from build123d import *

# Parameters (mm, degrees)
SKETCH1_W                = 188
SKETCH1_H                = 90
SKETCH1_R                = 3
BOSS_EXTRUDE1_DEPTH      = 2
BOSS_EXTRUDE2_DEPTH      = 31.5
BOSS_EXTRUDE2_DEPTH_BACK = 7
SKETCH2_W                = 14
SKETCH2_H                = 37


with BuildPart() as part:
    # Sketch1 → Boss-Extrude1 (new body)
    with BuildSketch(Plane(origin=(0, 0, 0), x_dir=(1, 0, 0), z_dir=(0, 1, 0))):
        Rectangle(SKETCH1_W, SKETCH1_H)
        with Locations(Location((-89, 37.75, 0), (0, 0, 270))):
            Circle(SKETCH1_R, mode=Mode.SUBTRACT)
        with Locations(Location((89, 37.75, 0), (0, 0, 270))):
            Circle(SKETCH1_R, mode=Mode.SUBTRACT)
        with Locations(Location((89, -37.75, 0), (0, 0, 270))):
            Circle(SKETCH1_R, mode=Mode.SUBTRACT)
        with Locations(Location((-89, -37.75, 0), (0, 0, 270))):
            Circle(SKETCH1_R, mode=Mode.SUBTRACT)
    extrude(amount=BOSS_EXTRUDE1_DEPTH)

    # Sketch2 → Boss-Extrude2 (add, two sides: drawn at the far end of the back side and taken through both)
    with BuildSketch(Plane(origin=(0, 2, 0), x_dir=(1, 0, 0), z_dir=(0, 1, 0)).offset(-BOSS_EXTRUDE2_DEPTH_BACK)):
        Polygon((-80, -28), (-80, -45), (80, -45), (80, 45), (-80, 45), (-80, 9), align=None)
        with Locations((-87, -9.5)):
            Rectangle(SKETCH2_W, SKETCH2_H)
    extrude(amount=BOSS_EXTRUDE2_DEPTH + BOSS_EXTRUDE2_DEPTH_BACK)


solid = part.part
CAD build for the part. Positions are in the model's coordinates, mm. A direction names the side the tool comes from. Give positions to 0.01 mm unless a question says otherwise; leave off trailing zeros. Order: outer loops, then holes, each group sorted by start corner. A loop starts at its lowest first (then second) coordinate and runs counter-clockwise, first axis right, second up. Notation, with made-up numbers: (-38.75, 64) -> (20.25, 64) arc R29 ccw to (20.25, 91) -> close; hole circle Ø10 at (38.25, 37.25). An arc over 180 degrees is marked (long way). Return JSON: item names as keys, results as strings.
Q1. Saw through at C-C (z = -11). Write the cut outline in (x, y).
Working result:
{"outline": "(-94, 0) -> (-80, 0) -> (-80, -5) -> (80, -5) -> (80, 0) -> (94, 0) -> (94, 2) -> (80, 2) -> (80, 33.5) -> (-80, 33.5) -> (-80, 2) -> (-94, 2) -> close"}
Q2. Saw through at B-B (z = 37.75). Write the cut outline in (x, y), then the cut area to 3 significant figures.
Working result:
{"outline": "(-94, 0) -> (-92, 0) -> (-92, 2) -> (-94, 2) -> close; (-86, 0) -> (-80, 0) -> (-80, -5) -> (80, -5) -> (80, 0) -> (86, 0) -> (86, 2) -> (80, 2) -> (80, 33.5) -> (-80, 33.5) -> (-80, 2) -> (-86, 2) -> close; (92, 0) -> (94, 0) -> (94, 2) -> (92, 2) -> close", "area": "6,190 mm²"}
Q3. Saw through at A-A (x = 89). Write the cut outline in (y, z), then the cut area to 3 significant figures.
Working result:
{"outline": "(0, -45) -> (2, -45) -> (2, -40.75) -> (0, -40.75) -> close; (0, -34.75) -> (2, -34.75) -> (2, 34.75) -> (0, 34.75) -> close; (0, 40.75) -> (2, 40.75) -> (2, 45) -> (0, 45) -> close", "area": "156 mm²"}
Q4. Flat gauge pins, fed straight in: pin 1 (8 mm diameter, centred on x = 89, z = 37.75, fed in from -Y); pin 2 (8 mm diameter, centred on x = 89, z = -37.75, fed in from +Y); pin 3 (4 mm diameter, centred on x = -84.5, y = 14.5, fed in from -Z); pin 4 (1.5 mm diameter, centred on y = 2.5, z = -20.5, fed in from -X). Where does each tip first touch, or does it go through?
Working result:
{"pin 1": "y = 0", "pin 2": "y = 2", "pin 3": "z = -9", "pin 4": "x = -94"}
Q5. Which spindle directions (+Z, -Z, +X, -X, +Y, -Y) get a long thin tool onto all of the face, cutting with end or side? Do faces 1 (the face through (-80, 18, 36)), 2 (the face through (87, 2, -1)), 3 (the face through (-87, 18, -9)). Say none if no direction does.
Working result:
{"face 1": "+Z, -X, +Y", "face 2": "+Z, -Z, +X, +Y", "face 3": "-Z, -X, +Y"}
Q6. Mould opens along Z. For faces 4 (the face through (80, 18, 1)), 5 (the face through (-87, 18, 28)), 6 (the face through (-91.93, 0.99, 37.1)) say: pulls with the +Z half, pulls with the -Z half, needs draft (parallel to the pull), parting line crosses it, or undercut.
Working result:
{"face 4": "needs draft", "face 5": "pulls with the +Z half", "face 6": "undercut"}
Q7. Saw through at D-D (y = 29.5). Write the cut outline in (x, z).
Working result:
{"outline": "(-94, -9) -> (-80, -9) -> (-80, -45) -> (80, -45) -> (80, 45) -> (-80, 45) -> (-80, 28) -> (-94, 28) -> close"}
Q8. Drill centre lines: line 1 (X direction, y = 0.6, z = -37.75); line 2 (X direction, y = 32.5, z = -7.5); line 3 (X direction, y = 8.5, z = -38.5). Where is each one in solid material? Low to high.
Working result:
{"line 1": "-94 to -92, -86 to 86, 92 to 94", "line 2": "-94 to 80", "line 3": "-80 to 80"}
